Can you work these out from the drawing? Everything is in mm from the part's minimum corner. A direction names the side the tool comes from. Coordinates: 2 decimals unless noted, no trailing zeros. Loops run counter-clockwise (first coordinate to the right, second up) from the corner with the lowest first, then second, coordinate; pieces in that order, holes last. Notation, with made-up numbers: (36.25, -11.75) - (55.25, -11.75) arc R13 ccw to (55.25, -6.75) - close; hole circle Ø1 at (58, -19). An arc over 180 degrees is marked (long way). Put each result on its own line as item: value. Start each with the question number.
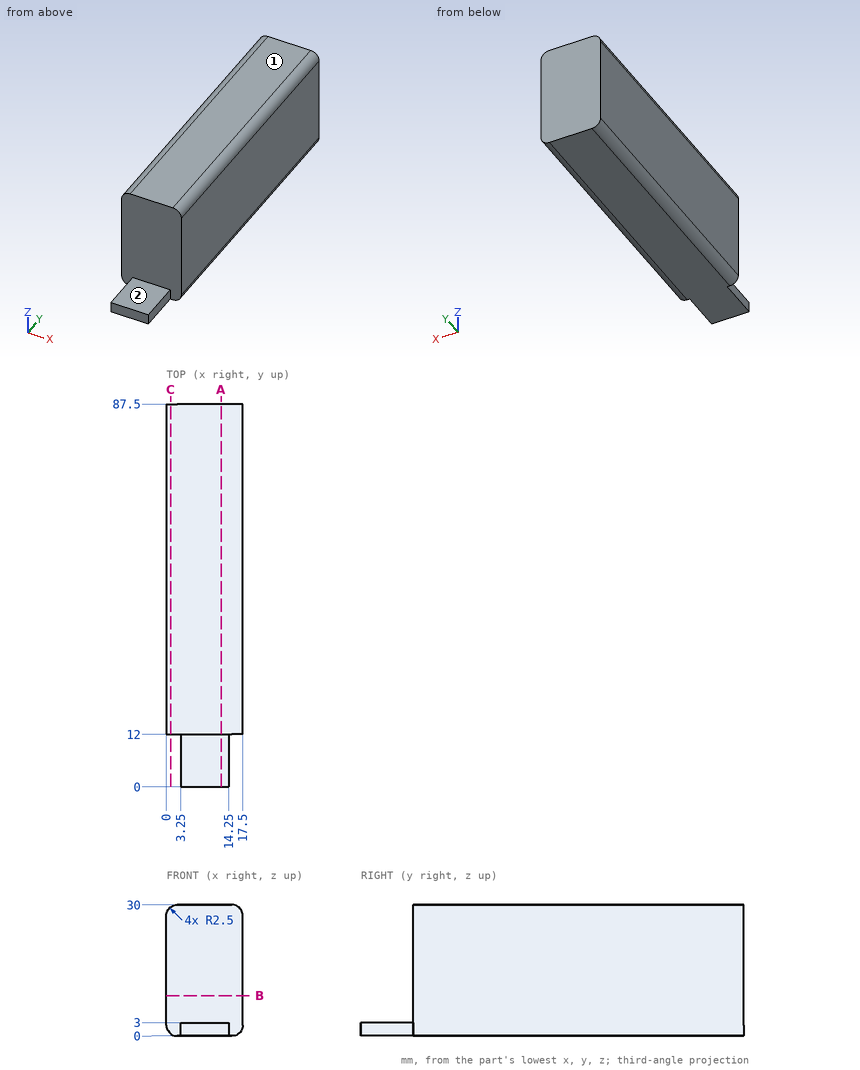
(1) For pin 1 Ø1.5 at (x, z) = (9.5, 9.5) entering from -Y; pin 2 Ø9 at (x, y) = (9, 8) entering from +Z; pin 3 Ø2.5 at (y, z) = (6, 1) entering from +X; pin 4 Ø0.9 at (y, z) = (3, 1) entering from -X, each with a flat end and sliding along its axis, tell me the tip position at first contact or that it passes through.
(2) I want a section at B-B on z = 9.25. List the corners of the cut face in (x, y) for me.
(3) Which directions (+Z, -Z, +X, -X, +Y, -Y) give clear straight access to the entire face, cutting with the end or side of a thin tool? Please do the marked faces 1 and 2.
(4) I want a section at C-C on x = 1. List the corners of the cut face in (y, z) for me, and give its area (3 significant figures).
(5) I want a section at A-A on x = 12.5. List the corners of the cut face in (y, z) for me.
(6) I need wall thicknesses on L1, parallel to Y at x = 10.25, z = 13.25; L2, parallel to Z at x = 17.25, y = 38.5; L3, parallel to Z at x = 1.5, y = 18.5. Which ranges of each line are inside material? Lowest first, please. Write a range as [from, to].
Answer sheet:
1. pin 1: stops at y = 12
1. pin 2: stops at z = 30
1. pin 3: stops at x = 14.25
1. pin 4: stops at x = 3.25
2. outline: (0, 12) - (17.5, 12) - (17.5, 87.5) - (0, 87.5) - close
3. face 1: +Z, +X, -X, +Y, -Y
3. face 2: +Z, +X, -X, -Y
4. outline: (12, 0.5) - (87.5, 0.5) - (87.5, 29.5) - (12, 29.5) - close
4. area: 2,190 mm^2
5. outline: (0, 0) - (87.5, 0) - (87.5, 30) - (12, 30) - (12, 3) - (0, 3) - close
6. L1: y = [12, 87.5]
6. L2: z = [1.41, 28.59]
6. L3: z = [0.21, 29.79]
